Source: CAD feature listing. Evaluate the final solid. Frame: model axes, mm. A direction names the side the tool comes from. Round coordinates to 2 decimals unless told otherwise and drop trailing zeros. Loops run counter-clockwise (first coordinate to the right, second up) from the corner with the lowest first, then second, coordinate; pieces in that order, holes last. Notation, with made-up numbers: M 79.25,17 L 103.25,17 A22 cw 103.25,52 Z; hole C 55.5,-24.75 d8. An arc over 180 degrees is marked long. Write each question's results on one line, items separated by ' | '. Start each with the question number.
1. Draft query along Z for faces 5 (the cylindrical face through (-113.461, 79.86, 56.996)), 6 (the cylindrical face through (59.94, 60.07, 2.64)), 7 (the flat face through (25, 19, 0)), 8 (the flat face through (-27.654, 122.395, -32.899)). Return one class per face: released by +Z, released by -Z, zero draft, split by the parting line, or undercut.
2. Ray query, line 1 (Z direction, x = 0, y = 97.75); line 2 (Z direction, x = 0, y = 118.75); line 3 (X direction, y = 80, z = -60). Return the intervals inside material, ascending.
3. Section D-D on y = 20. Output: boundary loops of the cut face in (x, z), and give its area (3 significant figures).
4. Section A-A on y = 120.5. Output: boundary loops of the cut face in (x, z), and give its area (3 significant figures).
5. Section B-B on z = -120. Output: boundary loops of the cut face in (x, y).
6. Contact query for flat-ended pins moving along their axis: pin 1 Ø4 at (x, y) = (39, 107) entering from +Z; pin 2 Ø8.5 at (x, z) = (40.5, -10) entering from -Y; pin 3 Ø1 at (x, z) = (-29, -76) entering from +Y. Output: stop coordinate, or through.
7. Section C-C on x = 104. Output: boundary loops of the cut face in (y, z).
8. Set-up query: faces 1 (the flat face through (-10, 90, 117)), 2 (the flat face through (-11, 115, -42)), 3 (the flat face through (-27.55, 122.4, 32.72)), 4 (the cylindrical face through (-27, 38, 0)). Return all of +Z, -Z, +X, -X, +Y, -Y with unobstructed straight access to the full face (end or side cutting, diameter ignored); none if empty.
from build123d import *

# Parameters (mm, degrees)
SKETCH4_W                               = 38.383060538
SKETCH4_H                               = 30
CUT_EXTRUDE1_DEPTH                      = 15
SKETCH5_W                               = 44.391966134
SKETCH5_H                               = 15
CUT_EXTRUDE2_DEPTH                      = 31
CBORE_FOR_M5_HEX_HEAD_BOLT1_D           = 20
CBORE_FOR_M5_HEX_HEAD_BOLT1_CBORE_D     = 30
CBORE_FOR_M5_HEX_HEAD_BOLT1_CBORE_DEPTH = 10
CIRPATTERN1_COUNT                       = 6
TAP_DRILL_FOR_M20X1_5_TAP1_D            = 18.5
CIRPATTERN2_COUNT                       = 2
CUT_EXTRUDE4_DEPTH                      = 30
FILLET1_R                               = 5
FILLET2_R                               = 10
SKETCH13_R                              = 8
CUT_EXTRUDE5_DEPTH                      = 126


with BuildPart() as part:
    # Sketch2 → Revolve1 (revolve)
    with BuildSketch(Plane.XY):
        Polygon((-20, 130), (-20, 110), (-15, 110), (-15, 0), (-30, 0), (-30, 50), (-60, 50), (-60, 70), (-150, 70), (-150, 100), (-50, 100), (-50, 130), align=None)
    revolve(axis=Axis((0, 0, 0), (0, 1, 0)))

    # Sketch4 → Cut-Extrude1 (cut)
    with BuildSketch(Plane(origin=(0, 100, 0), x_dir=(1, 0, 0), z_dir=(0, 1, 0))):
        Polygon((-49.681911326, -56.051594634), (-23.701149212, -71.051594634), (-4.509618943, -37.810889132), (-30.490381057, -22.810889132), align=None)
        with Locations((54.191530269, 0)):
            Rectangle(SKETCH4_W, SKETCH4_H)
        Polygon((-23.701149212, 71.051594634), (-49.681911326, 56.051594634), (-30.490381057, 22.810889132), (-4.509618943, 37.810889132), align=None)
    extrude(amount=CUT_EXTRUDE1_DEPTH, mode=Mode.SUBTRACT)

    # Sketch5 → Cut-Extrude2 (cut, through all)
    with BuildSketch(Plane(origin=(0, 100, 0), x_dir=(1, 0, 0), z_dir=(0, 1, 0))):
        Polygon((-46.191173595, -65.005459528), (-33.200792538, -72.505459528), (-11.004809472, -34.060889132), (-23.995190528, -26.560889132), align=None)
        with Locations((57.195983067, 0)):
            Rectangle(SKETCH5_W, SKETCH5_H)
        Polygon((-33.200792538, 72.505459528), (-46.191173595, 65.005459528), (-23.995190528, 26.560889132), (-11.004809472, 34.060889132), align=None)
    extrude(amount=CUT_EXTRUDE2_DEPTH, mode=Mode.SUBTRACT)

    # CBORE for M5 Hex Head Bolt1 (through all)
    with Locations(Plane(origin=(0, 100, 0), x_dir=(1, 0, 0), z_dir=(0, 1, 0))):
        with Locations((0, 120)):
            cbore_for_m5_hex_head_bolt1 = CounterBoreHole(CBORE_FOR_M5_HEX_HEAD_BOLT1_D / 2, CBORE_FOR_M5_HEX_HEAD_BOLT1_CBORE_D / 2, CBORE_FOR_M5_HEX_HEAD_BOLT1_CBORE_DEPTH)

    # CirPattern1: CBORE for M5 Hex Head Bolt1 ×6 about axis
    cirpattern1_axis = Axis((0, 0, 0), (0, 1, 0))
    for i in range(1, CIRPATTERN1_COUNT):
        add(cbore_for_m5_hex_head_bolt1.rotate(cirpattern1_axis, i * 360 / CIRPATTERN1_COUNT), mode=Mode.SUBTRACT)

    # Tap Drill for M20x1.5 Tap1 (through all)
    with Locations(Plane(origin=(0, 100, 0), x_dir=(1, 0, 0), z_dir=(0, 1, 0))):
        with Locations((0, 80)):
            tap_drill_for_m20x1_5_tap1 = Hole(TAP_DRILL_FOR_M20X1_5_TAP1_D / 2)

    # CirPattern2: Tap Drill for M20x1.5 Tap1 ×2 about axis
    cirpattern2_axis = Axis((0, 0, 0), (0, 1, 0))
    for i in range(1, CIRPATTERN2_COUNT):
        add(tap_drill_for_m20x1_5_tap1.rotate(cirpattern2_axis, i * 360 / CIRPATTERN2_COUNT), mode=Mode.SUBTRACT)

    # Sketch12 → Cut-Extrude4 (cut)
    with BuildSketch(Plane.XZ):
        with BuildLine():
            Line((-28.91366459, -8), (-25, -8))
            Line((-25, -8), (-25, 8))
            Line((-25, 8), (-28.91366459, 8))
            ThreePointArc((-28.91366459, 8), (-30, 0), (-28.91366459, -8))
        make_face()
        with BuildLine():
            Line((25, 8), (25, -8))
            Line((25, -8), (28.91366459, -8))
            ThreePointArc((28.91366459, -8), (30, 0), (28.91366459, 8))
            Line((28.91366459, 8), (25, 8))
        make_face()
    extrude(amount=-CUT_EXTRUDE4_DEPTH, mode=Mode.SUBTRACT)

    # Fillet1
    fillet1_edges = [part.edges().sort_by_distance(p)[0] for p in [
        (60, 70, 0),
        (60, 50, 0),
    ]]
    fillet(fillet1_edges, radius=FILLET1_R)

    # Fillet2
    fillet2_edges = [part.edges().sort_by_distance(p)[0] for p in [
        (30, 50, 0),
    ]]
    fillet(fillet2_edges, radius=FILLET2_R)

    # Sketch13 → Cut-Extrude5 (cut, through all)
    with BuildSketch(Plane(origin=(25, 0, 0), x_dir=(0, 0, -1), z_dir=(1, 0, 0))):
        with Locations((0, 30)):
            Circle(SKETCH13_R)
    cut_extrude5 = extrude(amount=CUT_EXTRUDE5_DEPTH, mode=Mode.SUBTRACT)

    # Mirror1: Cut-Extrude5 across plane
    add(cut_extrude5.mirror(Plane(origin=(0, 0, 0), x_dir=(0, 0, 1), z_dir=(1, 0, 0))), mode=Mode.SUBTRACT)


solid = part.part
Taken from the geometry:
1) face 5: undercut | face 6: split by the parting line | face 7: undercut | face 8: released by -Z
2) line 1: -150 to -135, -105 to -89.25, -70.75 to -15, 15 to 70.75, 89.25 to 105, 135 to 150 | line 2: -50 to -20, 20 to 50 | line 3: -137.48 to -113.92, -93.92 to 93.92, 113.92 to 137.48
3) outline: M -28.91,-8 A30 ccw 28.91,-8 L 25,-8 L 25,8 L 28.91,8 A30 ccw -28.91,8 L -25,8 L -25,-8 Z; hole C 0,0 d30 | area: 1,970 mm^2
4) outline: M -31.21,-39.06 L -24,-26.56 L -11,-34.06 L -18.22,-46.56 A50 ccw 49.43,-7.5 L 35,-7.5 L 35,7.5 L 49.43,7.5 A50 ccw -18.22,46.56 L -11,34.06 L -24,26.56 L -31.21,39.06 A50 ccw Z; hole C 0,0 d40 | area: 5,930 mm^2
5) outline: M -90,70 L -10,70 L -10,90 L -15,90 L -15,100 L -90,100 Z; M 10,70 L 90,70 L 90,100 L 15,100 L 15,90 L 10,90 Z
6) pin 1: z = 33.63 | pin 2: y = 49.67 | pin 3: y = 100
7) outline: M 70,-108.09 L 100,-108.09 L 100,-75 L 90,-75 L 90,-70 L 70,-70 Z; M 70,-50 L 90,-50 L 90,-45 L 100,-45 L 100,45 L 90,45 L 90,50 L 70,50 Z; M 70,70 L 90,70 L 90,75 L 100,75 L 100,108.09 L 70,108.09 Z
8) face 1: +Y | face 2: -X | face 3: +Z, +Y | face 4: -X, -Y
